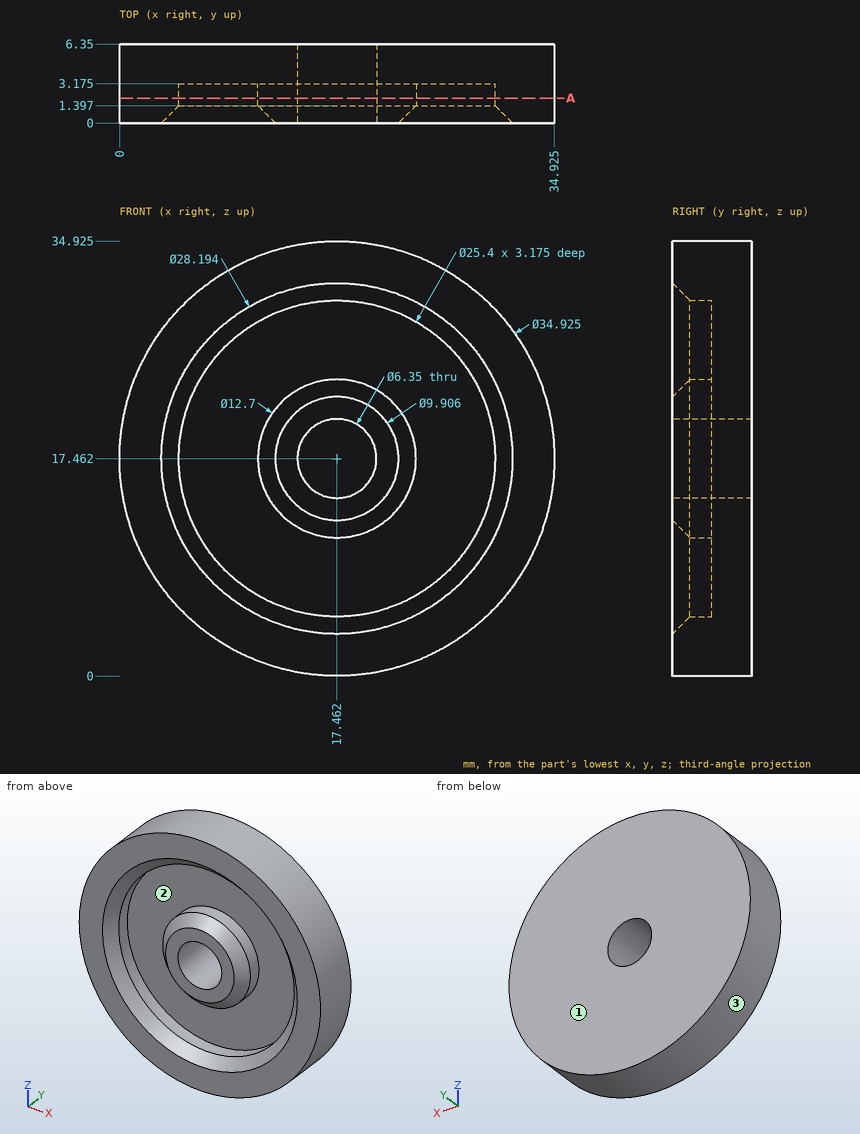
The drawing under review shows one solid part. Ordinate dimensions are in mm from its lowest x, y, z. Give positions to 0.01 mm unless a question says otherwise; leave off trailing zeros. Answer in a Markdown table with one row per item. Add a question column.
1. Draft analysis for pull direction Z (two halves, no side actions). For the marked faces 1, 2 and 3, state which applies: +Z half, -Z half, draft (parallel to the pull), parting line (faces both ways), or undercut.
2. Insertion check: P1, Ø1, axis at x = 12, y = 5, coming from the -Z side; P2, Ø2, axis at x = 6.5, y = 1.5, coming from the -Z side; P3, Ø1.5, axis at x = 20, y = 4, coming from the +Z side; P4, Ø15, axis at x = 17.46, z = 17.46, coming from the -Y side. Each pin has a flat end and moves straight along its axis. Give the tip position at first contact, or say it passes through.
3. We need section A-A on y = 2. State how many separate pieces and enclosed holes the cut face has.
4. Wall thickness on line 1 along Z through (x, y) = (22, 2) (1 decimal); line 2 along X through (y, z) = (4.75, 17.5) (1 decimal); line 3 along X through (y, z) = (5.75, 15.5) (1 decimal): over which ranges is each line inside the solid? List them lowest first. Write a range as [from, to].
Ans:
| question | item | result |
|---|---|---|
| 1 | face 1 | draft |
| 1 | face 2 | undercut |
| 1 | face 3 | parting line |
| 2 | P1 | stops at z = 0.72 |
| 2 | P2 | stops at z = 3.12 |
| 2 | P3 | stops at z = 34.83 |
| 2 | P4 | stops at y = 0 |
| 3 | separate pieces | 2 |
| 3 | enclosed holes | 2 |
| 4 | line 1 | z = [0.6, 5.6], [13, 21.9], [29.3, 34.3] |
| 4 | line 2 | x = [0, 14.3], [20.6, 34.9] |
| 4 | line 3 | x = [0.1, 15], [20, 34.8] |
